Here's how the part is built. I have some questions about the finished solid (model axes, mm). A direction names the side the tool comes from. Coordinates: 2 decimals unless noted, no trailing zeros. Write each loop counter-clockwise with the first axis right and the second up, starting at its lowest first coordinate (ties: lowest second). Pieces come first, ordered by that corner, then holes.
Item 1: If we mould it in two halves opening along X, with no side actions, what happens to faces 1 (the face through (655.175, 758.046, 1139.307)), 2 (the face through (445.44, 757.39, 1234.84)), 3 (the face through (563, 750, 1115.808))? For each: pulls with the +X half, pulls with the -X half, needs draft (parallel to the pull), parting line crosses it, or undercut.
Item 2: I'm going to push flat-ended pins straight in: P1, Ø2, axis at x = 534, y = 757.5, coming from the -Z side; P2, Ø3, axis at y = 758, z = 1253.5, coming from the -X side; P3, Ø1.5, axis at x = 468, y = 755, coming from the +Z side; P4, Ø2, axis at x = 578.88, z = 1215.5, coming from the -Y side. Where does each tip first touch, or does it pass through?
Item 3: For faces 4 (the face through (443.626, 750, 1232)), 5 (the face through (534.97, 758.05, 1259.31)), which set-ups out of +Z, -Z, +X, -X, +Y, -Y let a thin tool reach every point of the face, with its end or its side?
Item 4: Please list where these lines run through material, in increasing order: line 1 (X direction, y = 752.5, z = 1309.5); line 2 (Z direction, x = 573, y = 757.5); line 3 (Y direction, x = 543, z = 1225).
Item 5: I want a section at C-C (x = 554.5). Please give me the cut outline in (y, z).
Item 6: I want a section at B-B (z = 1190). Please give me the cut outline in (x, y), and give its area (3 significant figures).
Item 7: I want a section at A-A (x = 513). Please give me the cut outline in (y, z), and give its area (3 significant figures).
Item 8: I want a section at D-D (z = 1224). Please give me the cut outline in (x, y), and give its area (3 significant figures).
from build123d import *

# Parameters (mm, degrees)
BOSS_EXTRUDE1_DEPTH                                  = 12.7
FILLET1_R                                            = 6.35
CUT_EXTRUDE1_DEPTH                                   = 2.54
BOSS_EXTRUDE2_DEPTH                                  = 2.54
CSK_FOR_M3_HEX_SOCKET_COUNTERSUNK_CAP_SC_D           = 3.4
CSK_FOR_M3_HEX_SOCKET_COUNTERSUNK_CAP_SC_CSINK_D     = 6.72
CSK_FOR_M3_HEX_SOCKET_COUNTERSUNK_CAP_SC_CSINK_ANGLE = 90
CUT_EXTRUDE2_DEPTH                                   = 2.54
CSK_FOR_M3_HEX_SOCKET_COUNTERSUNK_CA_2_D             = 3.4
CSK_FOR_M3_HEX_SOCKET_COUNTERSUNK_CA_2_CSINK_D       = 6.72
CSK_FOR_M3_HEX_SOCKET_COUNTERSUNK_CA_2_CSINK_ANGLE   = 90


with BuildPart() as part:
    # Sketch2 → Boss-Extrude1 (new body)
    with BuildSketch(Plane(origin=(0, 759.298436, 0), x_dir=(-1, 0, 0), z_dir=(0, -1, 0))):
        with BuildLine():
            Line((-449.975603201, -1350.757525912), (-672.225603201, -1350.757525912))
            ThreePointArc((-672.225603201, -1350.757525912), (-676.715731261, -1348.897653973), (-678.575603201, -1344.407525912))
            Line((-678.575603201, -1344.407525912), (-678.575603201, -1122.157525912))
            ThreePointArc((-678.575603201, -1122.157525912), (-676.715731261, -1117.667397852), (-672.225603201, -1115.807525912))
            Line((-672.225603201, -1115.807525912), (-449.975603201, -1115.807525912))
            ThreePointArc((-449.975603201, -1115.807525912), (-445.48547514, -1117.667397852), (-443.625603201, -1122.157525912))
            Line((-443.625603201, -1122.157525912), (-443.625603201, -1344.407525912))
            ThreePointArc((-443.625603201, -1344.407525912), (-445.48547514, -1348.897653973), (-449.975603201, -1350.757525912))
        make_face()
    extrude(amount=BOSS_EXTRUDE1_DEPTH)

    # Fillet1
    fillet1_edges = [part.edges().sort_by_distance(p)[0] for p in [
        (678.575603201, 759.298436, 1233.282525912),
        (676.715731261, 759.298436, 1117.667397852),
        (561.100603201, 759.298436, 1115.807525912),
        (445.48547514, 759.298436, 1117.667397852),
        (443.625603201, 759.298436, 1233.282525912),
        (445.48547514, 759.298436, 1348.897653973),
        (561.100603201, 759.298436, 1350.757525912),
        (676.715731261, 759.298436, 1348.897653973),
    ]]
    fillet(fillet1_edges, radius=FILLET1_R)

    # Sketch4 → Cut-Extrude1 (cut)
    with BuildSketch(Plane(origin=(0, 759.298436, 0), x_dir=(1, 0, 0), z_dir=(0, 1, 0))):
        with BuildLine():
            Line((471.565603201, -1329.167525912), (650.635603201, -1329.167525912))
            ThreePointArc((650.635603201, -1329.167525912), (655.125731261, -1327.307653973), (656.985603201, -1322.817525912))
            Line((656.985603201, -1322.817525912), (656.985603201, -1143.747525912))
            ThreePointArc((656.985603201, -1143.747525912), (655.125731261, -1139.257397852), (650.635603201, -1137.397525912))
            Line((650.635603201, -1137.397525912), (471.565603201, -1137.397525912))
            ThreePointArc((471.565603201, -1137.397525912), (467.07547514, -1139.257397852), (465.215603201, -1143.747525912))
            Line((465.215603201, -1143.747525912), (465.215603201, -1322.817525912))
            ThreePointArc((465.215603201, -1322.817525912), (467.07547514, -1327.307653973), (471.565603201, -1329.167525912))
        make_face()
    extrude(amount=-CUT_EXTRUDE1_DEPTH, mode=Mode.SUBTRACT)

    # Sketch5 → Boss-Extrude2 (add)
    with BuildSketch(Plane(origin=(0, 756.758436, 0), x_dir=(1, 0, 0), z_dir=(0, 1, 0))):
        with BuildLine():
            Line((479.185603201, -1321.547525912), (643.015603201, -1321.547525912))
            ThreePointArc((643.015603201, -1321.547525912), (647.505731261, -1319.687653973), (649.365603201, -1315.197525912))
            Line((649.365603201, -1315.197525912), (649.365603201, -1151.367525912))
            ThreePointArc((649.365603201, -1151.367525912), (647.505731261, -1146.877397852), (643.015603201, -1145.017525912))
            Line((643.015603201, -1145.017525912), (479.185603201, -1145.017525912))
            ThreePointArc((479.185603201, -1145.017525912), (474.69547514, -1146.877397852), (472.835603201, -1151.367525912))
            Line((472.835603201, -1151.367525912), (472.835603201, -1315.197525912))
            ThreePointArc((472.835603201, -1315.197525912), (474.69547514, -1319.687653973), (479.185603201, -1321.547525912))
        make_face()
    extrude(amount=BOSS_EXTRUDE2_DEPTH)

    # CSK for M3 Hex Socket Countersunk Cap Sc (through all)
    with Locations(Plane.XZ.offset(-746.598436)):
        with Locations((484.900603201, 1157.082525912), (484.900603201, 1309.482525912), (637.300603201, 1309.482525912), (637.300603201, 1157.082525912)):
            CounterSinkHole(CSK_FOR_M3_HEX_SOCKET_COUNTERSUNK_CAP_SC_D / 2, CSK_FOR_M3_HEX_SOCKET_COUNTERSUNK_CAP_SC_CSINK_D / 2, counter_sink_angle=CSK_FOR_M3_HEX_SOCKET_COUNTERSUNK_CAP_SC_CSINK_ANGLE)

    # Sketch11 → Cut-Extrude2 (cut)
    with BuildSketch(Plane(origin=(0, 759.298436, 0), x_dir=(1, 0, 0), z_dir=(0, 1, 0))):
        with BuildLine():
            Line((539.510603201, -1261.222525912), (582.690603201, -1261.222525912))
            ThreePointArc((582.690603201, -1261.222525912), (587.180731261, -1259.362653973), (589.040603201, -1254.872525912))
            Line((589.040603201, -1254.872525912), (589.040603201, -1211.692525912))
            ThreePointArc((589.040603201, -1211.692525912), (587.180731261, -1207.202397852), (582.690603201, -1205.342525912))
            Line((582.690603201, -1205.342525912), (539.510603201, -1205.342525912))
            ThreePointArc((539.510603201, -1205.342525912), (535.02047514, -1207.202397852), (533.160603201, -1211.692525912))
            Line((533.160603201, -1211.692525912), (533.160603201, -1254.872525912))
            ThreePointArc((533.160603201, -1254.872525912), (535.02047514, -1259.362653973), (539.510603201, -1261.222525912))
        make_face()
    extrude(amount=-CUT_EXTRUDE2_DEPTH, mode=Mode.SUBTRACT)

    # CSK for M3 Hex Socket Countersunk Ca 2 (through all)
    with Locations(Plane.XZ.offset(-746.598436)):
        with Locations((578.880603201, 1215.502525912), (543.320603201, 1215.502525912), (543.320603201, 1251.062525912), (578.880603201, 1251.062525912)):
            CounterSinkHole(CSK_FOR_M3_HEX_SOCKET_COUNTERSUNK_CA_2_D / 2, CSK_FOR_M3_HEX_SOCKET_COUNTERSUNK_CA_2_CSINK_D / 2, counter_sink_angle=CSK_FOR_M3_HEX_SOCKET_COUNTERSUNK_CA_2_CSINK_ANGLE)


solid = part.part
Answer:
1. face 1: undercut
1. face 2: pulls with the -X half
1. face 3: needs draft
2. P1: stops at z = 1116.89
2. P2: stops at x = 444.71
2. P3: stops at z = 1350.62
2. P4: passes through
3. face 4: +Z, -Z, -X, +Y, -Y
3. face 5: +Y
4. line 1: x = 443.63 to 483.2, 486.6 to 635.6, 639 to 678.58
4. line 2: z = 1117.73 to 1137.4, 1145.02 to 1205.34, 1261.22 to 1321.55, 1329.17 to 1348.84
4. line 3: y = 746.6 to 756.76
5. outline: (746.6, 1115.81) - (752.95, 1115.81) arc R6.35 ccw to (759.3, 1122.16) - (759.3, 1137.4) - (756.76, 1137.4) - (756.76, 1145.02) - (759.3, 1145.02) - (759.3, 1205.34) - (756.76, 1205.34) - (756.76, 1261.22) - (759.3, 1261.22) - (759.3, 1321.55) - (756.76, 1321.55) - (756.76, 1329.17) - (759.3, 1329.17) - (759.3, 1344.41) arc R6.35 ccw to (752.95, 1350.76) - (746.6, 1350.76) - close
6. outline: (443.63, 746.6) - (678.58, 746.6) - (678.58, 752.95) arc R6.35 ccw to (672.23, 759.3) - (656.99, 759.3) - (656.99, 756.76) - (649.37, 756.76) - (649.37, 759.3) - (472.84, 759.3) - (472.84, 756.76) - (465.22, 756.76) - (465.22, 759.3) - (449.98, 759.3) arc R6.35 ccw to (443.63, 752.95) - close
6. area: 2,930 mm2
7. outline: (746.6, 1115.81) - (752.95, 1115.81) arc R6.35 ccw to (759.3, 1122.16) - (759.3, 1137.4) - (756.76, 1137.4) - (756.76, 1145.02) - (759.3, 1145.02) - (759.3, 1321.55) - (756.76, 1321.55) - (756.76, 1329.17) - (759.3, 1329.17) - (759.3, 1344.41) arc R6.35 ccw to (752.95, 1350.76) - (746.6, 1350.76) - close
7. area: 2,930 mm2
8. outline: (443.63, 746.6) - (678.58, 746.6) - (678.58, 752.95) arc R6.35 ccw to (672.23, 759.3) - (656.99, 759.3) - (656.99, 756.76) - (649.37, 756.76) - (649.37, 759.3) - (589.04, 759.3) - (589.04, 756.76) - (533.16, 756.76) - (533.16, 759.3) - (472.84, 759.3) - (472.84, 756.76) - (465.22, 756.76) - (465.22, 759.3) - (449.98, 759.3) arc R6.35 ccw to (443.63, 752.95) - close
8. area: 2,790 mm2
